from build123d import *

# Parameters (mm, degrees)
SKIZZE1_W                       = 325
SKIZZE1_H                       = 80
AUFSATZ_LINEAR_AUSTRAGEN1_DEPTH = 5
SKIZZE2_W                       = 100
SKIZZE2_H                       = 5
AUFSATZ_LINEAR_AUSTRAGEN3_DEPTH = 5
SKIZZE3_W                       = 5
SKIZZE3_H                       = 40
SCHNITT_LINEAR_AUSTRAGEN1_DEPTH = 335.738704066


with BuildPart() as part:
    # Skizze1 → Aufsatz-Linear austragen1 (new body)
    with BuildSketch(Plane.XY):
        with Locations((162.5, 40)):
            Rectangle(SKIZZE1_W, SKIZZE1_H)
    extrude(amount=AUFSATZ_LINEAR_AUSTRAGEN1_DEPTH)

    # Skizze2 → Aufsatz-Linear austragen3 (add, through all)
    with BuildSketch(Plane.XY.offset(5)):
        with Locations((162.5, -2.5)):
            Rectangle(SKIZZE2_W, SKIZZE2_H)
    extrude(amount=-AUFSATZ_LINEAR_AUSTRAGEN3_DEPTH)

    # Skizze3 → Schnitt-Linear austragen1 (cut, through all)
    with BuildSketch(Plane.XY.offset(5)):
        with Locations((2.5, 40)):
            Rectangle(SKIZZE3_W, SKIZZE3_H)
        with Locations((322.5, 40)):
            Rectangle(SKIZZE3_W, SKIZZE3_H)
    extrude(amount=-SCHNITT_LINEAR_AUSTRAGEN1_DEPTH, mode=Mode.SUBTRACT)


solid = part.part
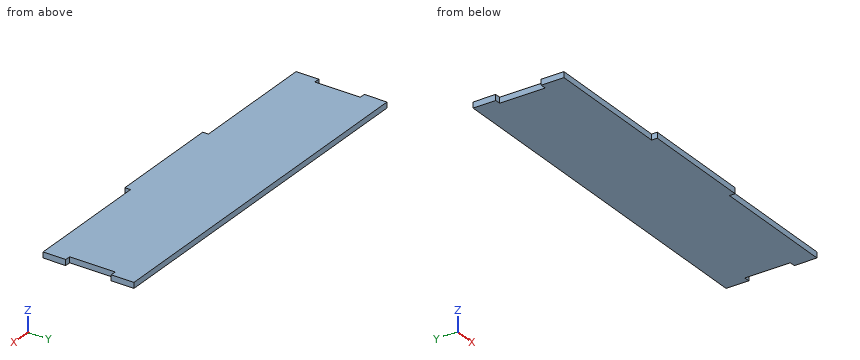
The listing builds one solid part. Answer for the finished solid, in the listing's coordinates (mm). Coordinates: 2 decimals unless noted, no trailing zeros. Loops run counter-clockwise (first coordinate to the right, second up) from the corner with the lowest first, then second, coordinate; pieces in that order, holes last.
1) Find section B-B on x = 94.5. Write down the section's boundary in (y, z), then the cut area to 3 significant figures.
2) Find the intervals of material crossed by L1, parallel to X at y = 23, z = 2; L2, parallel to Y at x = 27.5, z = 1.9, in increasing order.
3) Find section C-C on y = 49. Write down the section's boundary in (x, z), then the cut area to 4 significant figures.
4) Find section A-A on z = 3. Write down the section's boundary in (x, y), then the cut area to 3 significant figures.
5) Flat-ended cylindrical pins translate along their axes: pin 1 Ø2.5 at (x, z) = (81.5, 3.5) entering from -Y; pin 2 Ø1.5 at (y, z) = (-2, 2) entering from +X; pin 3 Ø2 at (y, z) = (57.5, 2.5) entering from -X. Find the tip coordinate at first contact, or state that the pin passes through.
Values:
1. outline: (0, 0) - (80, 0) - (80, 5) - (0, 5) - close
1. area: 400 mm2
2. L1: x = 5 to 320
2. L2: y = 0 to 80
3. outline: (5, 0) - (320, 0) - (320, 5) - (5, 5) - close
3. area: 1,575 mm2
4. outline: (0, 0) - (112.5, 0) - (112.5, -5) - (212.5, -5) - (212.5, 0) - (325, 0) - (325, 20) - (320, 20) - (320, 60) - (325, 60) - (325, 80) - (0, 80) - (0, 60) - (5, 60) - (5, 20) - (0, 20) - close
4. area: 26,100 mm2
5. pin 1: stops at y = 0
5. pin 2: stops at x = 212.5
5. pin 3: stops at x = 5
